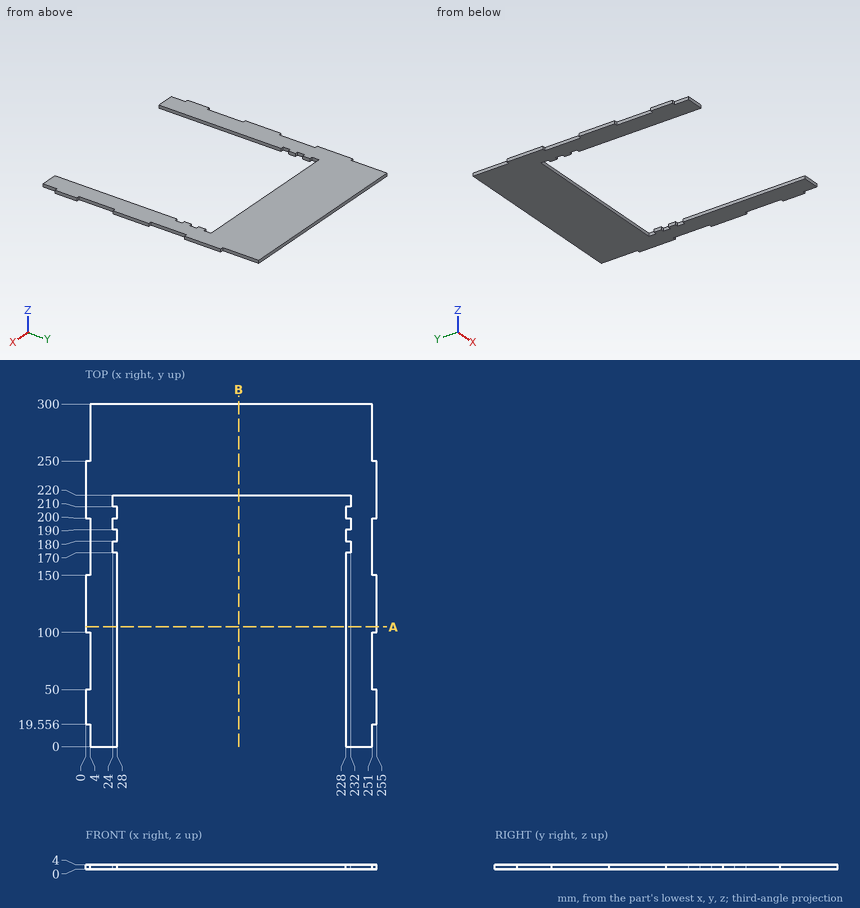
Geometry: see drawing. Coordinates: mm, zero at the bounding-box minimum. Coordinates: 2 decimals unless noted, no trailing zeros. Loops run counter-clockwise (first coordinate to the right, second up) from the corner with the lowest first, then second, coordinate; pieces in that order, holes last.
(1) Section A-A on y = 105. Return the cut outline in (x, z).
(2) Material intervals for probe 1 along Y at (x, z) = (230, 2.55); probe 2 along X at (y, z) = (166, 1.35); probe 3 along X at (y, z) = (31.5, 2.85), sorted ascending.
(3) Section B-B on x = 134. Return the cut outline in (y, z).
(4) First-contact query: pin 1 Ø2 at (y, z) = (270, 1) entering from +X; pin 2 Ø1.2 at (y, z) = (163.5, 2) entering from -X; pin 3 Ø1.2 at (x, z) = (1.5, 2.5) entering from -Y. Flat tips, straight axial feed; report the tip coordinate or a pass-through.
Data:
1. outline: (0, 0) - (28, 0) - (28, 4) - (0, 4) - close; (228, 0) - (255, 0) - (255, 4) - (228, 4) - close
2. probe 1: y = 0 to 170, 180 to 190, 200 to 210, 220 to 300
2. probe 2: x = 4 to 28, 228 to 251
2. probe 3: x = 0 to 28, 228 to 255
3. outline: (220, 0) - (300, 0) - (300, 4) - (220, 4) - close
4. pin 1: stops at x = 251
4. pin 2: stops at x = 4
4. pin 3: stops at y = 19.56
